from build123d import *

# Parameters (mm, degrees)
BOSS_EXTRUDE1_DEPTH   = 14
SKETCH1_W             = 3
SKETCH1_H             = 42.24
BOSS_EXTRUDE1_2_DEPTH = 14
SKETCH1_3_W           = 3
SKETCH1_3_H           = 16
SKETCH1_3_H_2         = 42.24
SKETCH1_3_W_2         = 81.7
SKETCH1_3_H_3         = 114.24
BOSS_EXTRUDE2_DEPTH   = 1
BOSS_EXTRUDE3_DEPTH   = 87.7
FILLET1_R             = 3
SKETCH3_W             = 2
SKETCH3_H             = 42.24
BOSS_EXTRUDE4_DEPTH   = 7
SKETCH4_W             = 16
SKETCH4_H             = 5.5
BOSS_EXTRUDE5_DEPTH   = 3


with BuildPart() as part:
    # Sketch1 → Boss-Extrude1 (new body)
    with BuildSketch(Plane(origin=(0, 0, 0), x_dir=(1, 0, 0), z_dir=(0, 1, 0))):
        Polygon((81.7, 0), (0, 0), (0, 20), (-3, 20), (-3, -3), (84.7, -3), (84.7, 117.24), (-3, 117.24), (-3, 94.24), (0, 94.24), (0, 114.24), (81.7, 114.24), align=None)
    extrude(amount=BOSS_EXTRUDE1_DEPTH)

    # Sketch1<3> → Boss-Extrude2 (add)
    with BuildSketch(Plane(origin=(0, 0, 0), x_dir=(1, 0, 0), z_dir=(0, 1, 0))):
        with Locations((-1.5, 86.24)):
            Rectangle(SKETCH1_3_W, SKETCH1_3_H)
        with Locations((-1.5, 57.12)):
            Rectangle(SKETCH1_3_W, SKETCH1_3_H_2)
        with Locations((-1.5, 28)):
            Rectangle(SKETCH1_3_W, SKETCH1_3_H)
        with Locations((40.85, 57.12)):
            Rectangle(SKETCH1_3_W_2, SKETCH1_3_H_3)
        Polygon((81.7, 0), (0, 0), (0, 20), (-3, 20), (-3, -3), (84.7, -3), (84.7, 117.24), (-3, 117.24), (-3, 94.24), (0, 94.24), (0, 114.24), (81.7, 114.24), align=None)
    extrude(amount=-BOSS_EXTRUDE2_DEPTH)



with BuildPart() as body_2:
    # Sketch1 → Boss-Extrude1 2 (new body)
    with BuildSketch(Plane(origin=(0, 0, 0), x_dir=(1, 0, 0), z_dir=(0, 1, 0))):
        with Locations((-1.5, 57.12)):
            Rectangle(SKETCH1_W, SKETCH1_H)
    extrude(amount=BOSS_EXTRUDE1_2_DEPTH)


with BuildPart() as part_1:
    add(part.part)

    add(body_2.part)  # Boss-Extrude3 merges body 2
    # Sketch2 → Boss-Extrude3 (add)
    with BuildSketch(Plane.ZY.offset(3)):
        Polygon((-117.24, -1), (-117.24, -7.301511381), (3, -1), (3, 0), (-117.24, 0), align=None)
    extrude(amount=-BOSS_EXTRUDE3_DEPTH)

    # Fillet1
    fillet1_edges = [part_1.edges().sort_by_distance(p)[0] for p in [
        (-3, 3.34924431, -117.24),
        (84.7, 3.34924431, -117.24),
        (84.7, 6.5, 3),
        (-3, 6.5, 3),
    ]]
    fillet(fillet1_edges, radius=FILLET1_R)

    # Sketch3 → Boss-Extrude4 (add)
    with BuildSketch(Plane(origin=(0, 0, 0), x_dir=(1, 0, 0), z_dir=(0, 1, 0))):
        with Locations((1, 57.12)):
            Rectangle(SKETCH3_W, SKETCH3_H)
        Polygon((2, 20), (2, 2), (79.7, 2), (79.7, 112.24), (2, 112.24), (2, 94.24), (0, 94.24), (0, 114.24), (81.7, 114.24), (81.7, 0), (0, 0), (0, 20), align=None)
    extrude(amount=BOSS_EXTRUDE4_DEPTH)

    # Sketch4 → Boss-Extrude5 (add)
    with BuildSketch(Plane.ZY.offset(3)):
        with Locations((-86.24, 11.25)):
            Rectangle(SKETCH4_W, SKETCH4_H)
        with Locations((-28, 11.25)):
            Rectangle(SKETCH4_W, SKETCH4_H)
    extrude(amount=-BOSS_EXTRUDE5_DEPTH)


solid = part_1.part
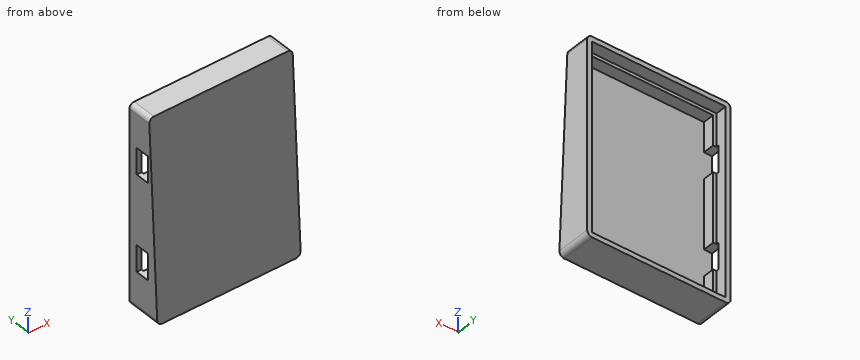
Could you check a few things on this model? Use its own coordinates, in mm. Coordinates: 2 decimals unless noted, no trailing zeros. Write each loop counter-clockwise with the first axis right and the second up, starting at its lowest first coordinate (ties: lowest second). Pieces come first, ordered by that corner, then holes. Notation, with made-up numbers: (25, -14.75) - (52, -14.75) arc R11 cw to (52, -6.75) - close; hole circle Ø11 at (83.25, 60.5). An arc over 180 degrees is marked (long way). Put each result on its own line as item: value. Start each with the question number.
Q1. Please list where these lines run through material, in increasing order: L1, parallel to X at y = 12.25, z = -94; L2, parallel to Z at x = 3.5, y = 5.5; L3, parallel to Z at x = 27.5, y = 9.5.
Q2. I want a section at D-D on z = -58. Write out the boundary of the cut face in (x, y).
Q3. I want a section at C-C on x = 16.5. Write out the boundary of the cut face in (y, z), plus the area to 3 significant figures.
Q4. I want a section at A-A on y = 1.5. Write out the boundary of the cut face in (x, z).
Q5. I want a section at B-B on y = 12.75. Write out the boundary of the cut face in (x, z), plus the area to 3 significant figures.
Q6. I'm going to push flat-ended pins straight in: P1, Ø2.5, axis at x = -1.5, z = -85.5, coming from the -Y side; P2, Ø2.5, axis at x = -1, z = -27.5, coming from the -Y side; P3, Ø25, axis at x = 20, z = -59.5, coming from the +Y side. Where does each tip first touch, or does it pass through?
Checks:
1. L1: -3 to 0, 81.7 to 84.7
1. L2: -117.24 to -112.24, -2 to 3
1. L3: -117.24 to -114.24, 0 to 3
2. outline: (-3, -4.2) - (84.7, -4.2) - (84.7, 14) - (81.7, 14) - (81.7, 7) - (79.7, 7) - (79.7, 0) - (2, 0) - (2, 7) - (0, 7) - (0, 14) - (-3, 14) - close
3. outline: (-7.3, -117.24) - (14, -117.24) - (14, -114.24) - (7, -114.24) - (7, -112.24) - (0, -112.24) - (0, -2) - (7, -2) - (7, 0) - (14, 0) - (14, 3) - (-1, 3) - close
3. area: 611 mm²
4. outline: (-3, -114.24) arc R3 ccw to (0, -117.24) - (81.7, -117.24) arc R3 ccw to (84.7, -114.24) - (84.7, 0) arc R3 ccw to (81.7, 3) - (0, 3) arc R3 ccw to (-3, 0) - (-3, -20) - (2, -20) - (2, -2) - (79.7, -2) - (79.7, -112.24) - (2, -112.24) - (2, -94.24) - (-3, -94.24) - close; (-3, -78.24) - (2, -78.24) - (2, -36) - (-3, -36) - close
5. outline: (-3, -114.24) arc R3 ccw to (0, -117.24) - (81.7, -117.24) arc R3 ccw to (84.7, -114.24) - (84.7, 0) arc R3 ccw to (81.7, 3) - (0, 3) arc R3 ccw to (-3, 0) - close; hole (0, -114.24) - (81.7, -114.24) - (81.7, 0) - (0, 0) - close
5. area: 1,200 mm²
6. P1: y = -5.7
6. P2: y = -2.66
6. P3: y = 0
